Could you check a few things on this model? Use its own coordinates, in mm. Round coordinates to 2 decimals unless told otherwise and drop trailing zeros. Loops run counter-clockwise (first coordinate to the right, second up) from the corner with the lowest first, then second, coordinate; pieces in that order, holes last. Notation, with made-up numbers: (82.25, 28.25) -> (129.25, 28.25) arc R10 ccw to (129.25, 36.25) -> close; hole circle Ø11 at (53, -22.75). An arc over 180 degrees is marked (long way). One line per item, written item: value.
from build123d import *

# Parameters (mm, degrees)
F0_R     = 9.8679
F0_R_2   = 11.25
F1_DEPTH = 7.62
F2_R     = 7.62


with BuildPart() as f1:
    # F0 (on Top) → F1 (new body)
    with BuildSketch(Plane.XY):
        with BuildLine():
            ThreePointArc((-43.9675390459, -18.2733148979), (-24.0769783095, -20.7336914411), (-5.6897763655, -12.7588144007))
            ThreePointArc((-5.6897763655, -12.7588144007), (-11.3636627485, -8.1257657448), (-13.9131894177, -1.2585945443))
            ThreePointArc((-13.9131894177, -1.2585945443), (-17.7883649195, -6.3661757884), (-23.5779527058, -3.6120798208))
            ThreePointArc((-23.5779527058, -3.6120798208), (-23.9117664703, -3.0016925054), (-24.27850376, -2.4105004347))
            ThreePointArc((-24.27850376, -2.4105004347), (-26.3622058351, 0.0187882898), (-28.9870638751, 1.8500114644))
            ThreePointArc((-28.9870638751, 1.8500114644), (-31.9863775374, 2.9668711691), (-35.1696654297, 3.2984375125))
            ThreePointArc((-35.1696654297, 3.2984375125), (-36.9929388731, 3.125210966), (-38.772336885, 2.6915334348))
            ThreePointArc((-38.772336885, 2.6915334348), (-40.0568325476, 2.2001090277), (-41.2806580353, 1.5726711973))
            ThreePointArc((-41.2806580353, 1.5726711973), (-42.7921593571, 0.5384095089), (-44.1391793855, -0.7025056892))
            ThreePointArc((-44.1391793855, -0.7025056892), (-47.5826237378, -9.5223858919), (-43.9675390459, -18.2733148979))
        make_face()
        with Locations((-36.0358898416, -8.480387548)):
            Circle(F0_R, mode=Mode.SUBTRACT)
        with BuildLine():
            ThreePointArc((8.0465695573, -11.4198782113), (12.4010377936, -6.4323527299), (13.97, 0))
            ThreePointArc((13.97, 0), (13.9510735733, 0.7269430186), (13.8943455759, 1.4519163259))
            ThreePointArc((13.8943455759, 1.4519163259), (11.3636627485, 8.1257657448), (5.8666198604, 12.6784727555))
            ThreePointArc((5.8666198604, 12.6784727555), (-1.355288186, 13.9041034926), (-8.2045692104, 11.3068980747))
            ThreePointArc((-8.2045692104, 11.3068980747), (-12.7189509344, 5.7783377478), (-13.9131894177, -1.2585945443))
            ThreePointArc((-13.9131894177, -1.2585945443), (-11.3636627485, -8.1257657448), (-5.6897763655, -12.7588144007))
            ThreePointArc((-5.6897763655, -12.7588144007), (1.355288186, -13.9041034926), (8.0465695573, -11.4198782113))
        make_face()
        Circle(F0_R_2, mode=Mode.SUBTRACT)
        with BuildLine():
            ThreePointArc((-43.025617844, 8.8228840299), (-46.2565836802, 4.3728136122), (-44.1391793855, -0.7025056892))
            ThreePointArc((-44.1391793855, -0.7025056892), (-42.7921593571, 0.5384095089), (-41.2806580353, 1.5726711973))
            ThreePointArc((-41.2806580353, 1.5726711973), (-41.7197337386, 3.26892729), (-41.8789534473, 5.0138402649))
            ThreePointArc((-41.8789534473, 5.0138402649), (-42.7619749641, 6.8251340993), (-43.025617844, 8.8228840299))
        make_face()
        with BuildLine():
            ThreePointArc((-32.4148590407, 15.8445106758), (-39.2100586679, 12.2320065578), (-41.8789534473, 5.0138402649))
            ThreePointArc((-41.8789534473, 5.0138402649), (-40.5095024441, 3.6067356872), (-38.772336885, 2.6915334348))
            ThreePointArc((-38.772336885, 2.6915334348), (-36.9929388731, 3.125210966), (-35.1696654297, 3.2984375125))
            ThreePointArc((-35.1696654297, 3.2984375125), (-35.4953325875, 9.945426089), (-32.4148590407, 15.8445106758))
        make_face()
        with BuildLine():
            ThreePointArc((-41.8789534473, 5.0138402649), (-41.7197337386, 3.26892729), (-41.2806580353, 1.5726711973))
            ThreePointArc((-41.2806580353, 1.5726711973), (-40.0568325476, 2.2001090277), (-38.772336885, 2.6915334348))
            ThreePointArc((-38.772336885, 2.6915334348), (-40.5095024441, 3.6067356872), (-41.8789534473, 5.0138402649))
        make_face()
        with BuildLine():
            ThreePointArc((-35.1696654297, 3.2984375125), (-31.9863775374, 2.9668711691), (-28.9870638751, 1.8500114644))
            ThreePointArc((-28.9870638751, 1.8500114644), (-28.3049856869, 9.8245411614), (-22.2233339706, 15.0276043883))
            ThreePointArc((-22.2233339706, 15.0276043883), (-31.268583607, 12.0020163498), (-35.1696654297, 3.2984375125))
        make_face()
        with BuildLine():
            ThreePointArc((-28.9870638751, 1.8500114644), (-26.3622058351, 0.0187882898), (-24.27850376, -2.4105004347))
            ThreePointArc((-24.27850376, -2.4105004347), (-22.3038787795, 3.2440665901), (-16.8522933059, 5.7246890677))
            ThreePointArc((-16.8522933059, 5.7246890677), (-23.6023200247, 5.925256444), (-28.9870638751, 1.8500114644))
        make_face()
        with BuildLine():
            ThreePointArc((-8.2045692104, 11.3068980747), (-1.355288186, 13.9041034926), (5.8666198604, 12.6784727555))
            ThreePointArc((5.8666198604, 12.6784727555), (3.3809125021, 18.5882638063), (8.6608234676, 22.2251459229))
            ThreePointArc((8.6608234676, 22.2251459229), (9.3563412711, 22.2090434653), (10.0516972677, 22.2310512394))
            ThreePointArc((10.0516972677, 22.2310512394), (13.1973740538, 22.8209458081), (16.095688863, 24.1785279647))
            ThreePointArc((16.095688863, 24.1785279647), (18.5625745709, 26.2175799379), (20.4413633934, 28.8086049485))
            ThreePointArc((20.4413633934, 28.8086049485), (21.2029815253, 30.4742193418), (21.7171047722, 32.2320619891))
            ThreePointArc((21.7171047722, 32.2320619891), (21.9337665829, 33.5901800675), (22.0023022263, 34.9637629448))
            ThreePointArc((22.0023022263, 34.9637629448), (21.8623559909, 36.7898923316), (21.4612019196, 38.5769034946))
            ThreePointArc((21.4612019196, 38.5769034946), (15.5446837819, 45.9689538816), (6.15861461, 47.2136632046))
            ThreePointArc((6.15861461, 47.2136632046), (-5.9174143474, 31.218120583), (-8.2045692104, 11.3068980747))
        make_face()
        with Locations((10.6737138703, 35.4481898248)):
            Circle(F0_R, mode=Mode.SUBTRACT)
        with BuildLine():
            ThreePointArc((13.8943455759, 1.4519163259), (13.9510735733, 0.7269430186), (13.97, 0))
            ThreePointArc((13.97, 0), (12.4010377936, -6.4323527299), (8.0465695573, -11.4198782113))
            ThreePointArc((8.0465695573, -11.4198782113), (14.4074524174, -12.2220880179), (14.9171292382, -18.6130661021))
            ThreePointArc((14.9171292382, -18.6130661021), (14.5554251992, -19.2073509599), (14.2268064923, -19.8205508047))
            ThreePointArc((14.2268064923, -19.8205508047), (13.1648317813, -22.8397340979), (12.891375012, -26.0285394291))
            ThreePointArc((12.891375012, -26.0285394291), (13.4238029666, -29.184451107), (14.7283020363, -32.1070424609))
            ThreePointArc((14.7283020363, -32.1070424609), (15.7899573478, -33.5994303078), (17.0552321128, -34.9235954239))
            ThreePointArc((17.0552321128, -34.9235954239), (18.1230659647, -35.7902890953), (19.278355809, -36.5364341421))
            ThreePointArc((19.278355809, -36.5364341421), (20.9298033662, -37.3283018405), (22.6779774659, -37.8743978054))
            ThreePointArc((22.6779774659, -37.8743978054), (32.0379399559, -36.4465679897), (37.8089244359, -28.9403483066))
            ThreePointArc((37.8089244359, -28.9403483066), (29.994392657, -10.4844291419), (13.8943455759, 1.4519163259))
        make_face()
        with Locations((25.3621759713, -26.9678022769)):
            Circle(F0_R, mode=Mode.SUBTRACT)
        with BuildLine():
            ThreePointArc((29.1536506265, 32.8498360514), (26.9152595143, 37.8729697533), (21.4612019196, 38.5769034946))
            ThreePointArc((21.4612019196, 38.5769034946), (21.8623559909, 36.7898923316), (22.0023022263, 34.9637629448))
            ThreePointArc((22.0023022263, 34.9637629448), (23.6908409456, 34.4958856118), (25.2815897635, 33.7613174369))
            ThreePointArc((25.2815897635, 33.7613174369), (27.2917269962, 33.6203895852), (29.1536506265, 32.8498360514))
        make_face()
        with BuildLine():
            ThreePointArc((21.7171047722, 32.2320619891), (21.2029815253, 30.4742193418), (20.4413633934, 28.8086049485))
            ThreePointArc((20.4413633934, 28.8086049485), (26.3606579383, 25.7671466921), (29.9291782762, 20.1498360514))
            ThreePointArc((29.9291782762, 20.1498360514), (30.1982577523, 27.8409036114), (25.2815897635, 33.7613174369))
            ThreePointArc((25.2815897635, 33.7613174369), (23.3782759519, 33.2788903677), (21.7171047722, 32.2320619891))
        make_face()
        with BuildLine():
            ThreePointArc((20.4413633934, 28.8086049485), (18.5625745709, 26.2175799379), (16.095688863, 24.1785279647))
            ThreePointArc((16.095688863, 24.1785279647), (22.6607950698, 19.6005660779), (24.1259541436, 11.7321695811))
            ThreePointArc((24.1259541436, 11.7321695811), (26.028342859, 21.0783795691), (20.4413633934, 28.8086049485))
        make_face()
        with BuildLine():
            ThreePointArc((16.095688863, 24.1785279647), (13.1973740538, 22.8209458081), (10.0516972677, 22.2310512394))
            ThreePointArc((10.0516972677, 22.2310512394), (13.9613834684, 17.6936923309), (13.3838728144, 11.7321695811))
            ThreePointArc((13.3838728144, 11.7321695811), (16.9325826168, 17.4775805077), (16.095688863, 24.1785279647))
        make_face()
        with BuildLine():
            ThreePointArc((25.2815897635, 33.7613174369), (23.6908409456, 34.4958856118), (22.0023022263, 34.9637629448))
            ThreePointArc((22.0023022263, 34.9637629448), (21.9337665829, 33.5901800675), (21.7171047722, 32.2320619891))
            ThreePointArc((21.7171047722, 32.2320619891), (23.3782759519, 33.2788903677), (25.2815897635, 33.7613174369))
        make_face()
        with BuildLine():
            ThreePointArc((12.891375012, -26.0285394291), (13.1648317813, -22.8397340979), (14.2268064923, -19.8205508047))
            ThreePointArc((14.2268064923, -19.8205508047), (8.3424953112, -20.937758921), (3.4684204916, -17.4568586488))
            ThreePointArc((3.4684204916, -17.4568586488), (6.6697374079, -23.4028369517), (12.891375012, -26.0285394291))
        make_face()
        with BuildLine():
            ThreePointArc((14.7283020363, -32.1070424609), (13.4238029666, -29.184451107), (12.891375012, -26.0285394291))
            ThreePointArc((12.891375012, -26.0285394291), (5.6441906172, -29.4251072393), (-1.902620173, -26.7597739695))
            ThreePointArc((-1.902620173, -26.7597739695), (5.240240748, -33.0803959189), (14.7283020363, -32.1070424609))
        make_face()
        with BuildLine():
            ThreePointArc((13.8719672174, -41.6727200814), (19.341324166, -42.2457833654), (22.6779774659, -37.8743978054))
            ThreePointArc((22.6779774659, -37.8743978054), (20.9298033662, -37.3283018405), (19.278355809, -36.5364341421))
            ThreePointArc((19.278355809, -36.5364341421), (18.028892793, -37.7648129018), (16.5973636838, -38.7751577017))
            ThreePointArc((16.5973636838, -38.7751577017), (15.4702479678, -40.4455236845), (13.8719672174, -41.6727200814))
        make_face()
        with BuildLine():
            ThreePointArc((2.4856807646, -35.9943467273), (9.0118009156, -40.0729101692), (16.5973636838, -38.7751577017))
            ThreePointArc((16.5973636838, -38.7751577017), (17.1312264922, -36.8856260549), (17.0552321128, -34.9235954239))
            ThreePointArc((17.0552321128, -34.9235954239), (15.7899573478, -33.5994303078), (14.7283020363, -32.1070424609))
            ThreePointArc((14.7283020363, -32.1070424609), (9.1346746492, -35.7125727811), (2.4856807646, -35.9943467273))
        make_face()
        with BuildLine():
            ThreePointArc((16.5973636838, -38.7751577017), (18.028892793, -37.7648129018), (19.278355809, -36.5364341421))
            ThreePointArc((19.278355809, -36.5364341421), (18.1230659647, -35.7902890953), (17.0552321128, -34.9235954239))
            ThreePointArc((17.0552321128, -34.9235954239), (17.1312264922, -36.8856260549), (16.5973636838, -38.7751577017))
        make_face()
    extrude(amount=F1_DEPTH)

    # F2
    f2_edges = [f1.edges().sort_by_distance(p)[0] for p in [
        (37.808924, -28.940348, 3.81),
        (6.158615, 47.213663, 3.81),
        (-43.967539, -18.273315, 3.81),
    ]]
    fillet(f2_edges, radius=F2_R)


solid = f1.part
(1) If I drill on L1, parallel to Y at x = -27, z = 6; L2, parallel to Y at x = 28, z = 4.5; L3, parallel to X at y = -7, z = 6.75, over which ranges is the centre line in solid material (lowest first)?
Recorded:
L1: -21.04 to -12.45, -4.51 to 4.07, 11.79 to 14.48
L2: -37.98 to -36.48, -17.46 to -8.15, 23.95 to 31.58, 33.41 to 36.81
L3: -47.35 to -45.79, -26.28 to -8.81, 8.81 to 26.89
(2) If we section it at A-A, the plane x = -40.5: Please give me the cut outline in (y, z), then the cut area to 3 significant figures.
Recorded:
outline: (-19.5, 0) -> (-17.28, 0) -> (-17.28, 7.62) -> (-19.5, 7.62) -> close; (0.32, 0) -> (10.4, 0) -> (10.4, 7.62) -> (0.32, 7.62) -> close
area: 93.8 mm²
(3) If we section it at B-B, the plane z = 3.5: Give the number of separate pieces and of enclosed holes in the cut face, then the cut area to 3 significant figures.
Recorded:
separate pieces: 1
enclosed holes: 4
area: 1,910 mm²
(4) I'm going to push flat-ended pins straight in: pin 1 Ø10 at (x, y) = (-13.5, 35) entering from +Z; pin 2 Ø3 at (x, z) = (13, 1) entering from +Y; pin 3 Ø4 at (x, z) = (8, 6) entering from -Y. Where does each tip first touch, or does it pass through?
Recorded:
pin 1: through
pin 2: y = 47.42
pin 3: y = -40.22
(5) Thinking about a two-plate mould opening in X: for faces 1 (the face through (5, -33, 4)), 2 (the face through (-5, -11, 7.62)), 3 (the face through (16.91, 17.38, 3.76)), which applies, released by +X, released by -X, zero draft, split by the parting line, or undercut?
Recorded:
face 1: undercut
face 2: zero draft
face 3: undercut
